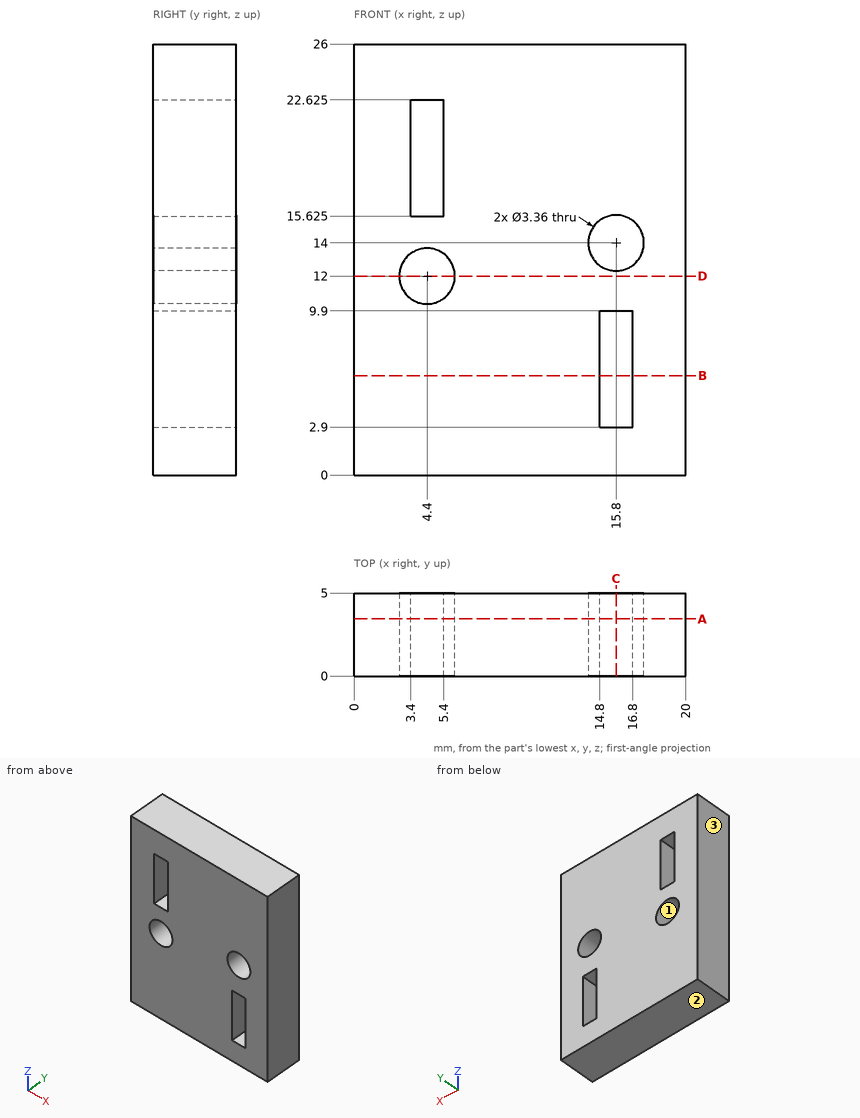
Geometry: see drawing. Coordinates: mm, zero at the bounding-box minimum. Coordinates: 2 decimals unless noted, no trailing zeros. Loops run counter-clockwise (first coordinate to the right, second up) from the corner with the lowest first, then second, coordinate; pieces in that order, holes last.
(1) Section A-A on y = 3.45. Return the cut outline in (x, z) (3 decimals).
(2) Pull-direction query (X, two-part tool) for the marked faces 1, 2 and 3; classes: released by +X, released by -X, zero draft, split by the parting line, or undercut.
(3) Section B-B on z = 6. Return the cut outline in (x, y).
(4) Section C-C on x = 15.8. Return the cut outline in (y, z).
(5) Material intervals for probe 1 along Z at (x, y) = (4.4, 1.8) (3 decimals); probe 2 along X at (y, z) = (4.4, 17.25); probe 3 along Z at (x, y) = (16.75, 1.25), sorted ascending.
(6) Section D-D on z = 12. Return the cut outline in (x, y).
Data:
1. outline: (0, 0) - (20, 0) - (20, 26) - (0, 26) - close; hole circle Ø3.36 at (4.4, 12); hole (3.4, 15.625) - (5.4, 15.625) - (5.4, 22.625) - (3.4, 22.625) - close; hole circle Ø3.36 at (15.8, 14); hole (14.8, 2.9) - (16.8, 2.9) - (16.8, 9.9) - (14.8, 9.9) - close
2. face 1: undercut
2. face 2: zero draft
2. face 3: released by -X
3. outline: (0, 0) - (14.8, 0) - (14.8, 5) - (0, 5) - close; (16.8, 0) - (20, 0) - (20, 5) - (16.8, 5) - close
4. outline: (0, 0) - (5, 0) - (5, 2.9) - (0, 2.9) - close; (0, 9.9) - (5, 9.9) - (5, 12.32) - (0, 12.32) - close; (0, 15.68) - (5, 15.68) - (5, 26) - (0, 26) - close
5. probe 1: z = 0 to 10.32, 13.68 to 15.625, 22.625 to 26
5. probe 2: x = 0 to 3.4, 5.4 to 20
5. probe 3: z = 0 to 2.9, 9.9 to 12.61, 15.39 to 26
6. outline: (0, 0) - (2.72, 0) - (2.72, 5) - (0, 5) - close; (6.08, 0) - (20, 0) - (20, 5) - (6.08, 5) - close
